Autodesk Inventor part; units mm, degrees
ref_plane "YZ Plane" through (0, 0, 0) normal (1, 0, 0) x (0, 1, 0)
ref_plane "XZ Plane" through (0, 0, 0) normal (0, 1, 0) x (-1, 0, 0)
ref_plane "XY Plane" through (0, 0, 0) normal (0, 0, 1) x (1, 0, 0)
sketch "Sketch1" plane through (0, 0, 0) normal (0, 1, 0) x (-1, 0, 0)
  line L0 (0, 0) -> (-88.9, 0)
  line L1 (-88.9, -114.3) -> (-88.9, -317.5)
  line L2 (-88.9, -431.8) -> (0, -431.8)
  line L3 (0, -431.8) -> (0, 0)
  line L4 (-88.9, 0) -> (-165.1, 0)
  line L5 (-165.1, 0) -> (-165.1, -114.3)
  line L6 (-165.1, -114.3) -> (-88.9, -114.3)
  line L7 (-88.9, -114.3) -> (-88.9, 0)
  line L8 (-88.9, -431.8) -> (-165.1, -431.8)
  line L9 (-165.1, -431.8) -> (-165.1, -317.5)
  line L10 (-165.1, -317.5) -> (-88.9, -317.5)
  line L11 (-88.9, -317.5) -> (-88.9, -431.8)
  line L12 (-88.9, -374.65) -> (-139.7, -374.65) construction
  line L13 (-88.9, -58.8342) -> (-139.7, -58.8342) construction
  circle A0 centre (-139.7, -58.8342) radius 7.9375
  circle A1 centre (-139.7, -374.65) radius 7.9375
  dimension "d0" = 88.9
  dimension "d1" = 431.8
  dimension "d2" = 76.2
  dimension "d3" = 114.3
  dimension "d4" = 76.2
  dimension "d5" = 114.3
  dimension "d6" = 50.8
  dimension "d7" = 15.875
  dimension "d8" = 15.875
extrude "Extrusion1" add sketch "Sketch1" along normal blind 6.35
sketch "Sketch8" plane through (0, 6.35, 0) normal (0, 1, 0) x (1, 0, 0)
  circle A0 centre (139.7, 58.8342) radius 7.9375
  circle A1 centre (139.7, 374.65) radius 7.9375
  line L0 (88.9, 317.5) -> (165.1, 317.5)
  line L1 (165.1, 317.5) -> (165.1, 431.8)
  line L2 (165.1, 431.8) -> (0, 431.8)
  line L3 (0, 431.8) -> (0, 0)
  line L4 (0, 0) -> (165.1, 0)
  line L5 (165.1, 0) -> (165.1, 114.3)
  line L6 (165.1, 114.3) -> (88.9, 114.3)
  line L7 (88.9, 114.3) -> (88.9, 317.5)
  line L8 (165.1, 0) -> (88.9, 0)
  line L9 (88.9, 0) -> (88.9, 3.175)
  line L10 (88.9, 3.175) -> (165.1, 3.175)
  line L11 (165.1, 3.175) -> (165.1, 0)
  line L12 (165.1, 114.3) -> (88.9, 114.3)
  line L13 (88.9, 114.3) -> (88.9, 111.125)
  line L14 (88.9, 111.125) -> (165.1, 111.125)
  line L15 (165.1, 111.125) -> (165.1, 114.3)
  line L16 (88.9, 114.3) -> (88.9, 317.5)
  line L17 (165.1, 317.5) -> (88.9, 317.5)
  line L18 (88.9, 317.5) -> (88.9, 320.675)
  line L19 (88.9, 320.675) -> (165.1, 320.675)
  line L20 (165.1, 320.675) -> (165.1, 317.5)
  line L21 (165.1, 431.8) -> (88.9, 431.8)
  line L22 (88.9, 431.8) -> (88.9, 428.625)
  line L23 (88.9, 428.625) -> (165.1, 428.625)
  line L24 (165.1, 428.625) -> (165.1, 431.8)
  dimension "d27" = 3.175
  dimension "d28" = 3.175
  dimension "d29" = 3.175
  dimension "d30" = 3.175
extrude "Extrusion7" add sketch "Sketch8" along normal blind 82.55 contours L18 L19 L1 L0 | L6 L5 L14 L13 | L23 L22 L2 L1 | L5 L4 L9 L10
sketch "Sketch9" plane through (165.1, 6.35, -3.175) normal (0, 0, -1) x (-1, 0, 0)
  line L0 (76.2, 0) -> (0, 0)
  line L1 (76.2, 0) -> (76.2, 82.55)
  line L2 (0, 82.55) -> (76.2, 82.55)
  line L3 (0, 0) -> (0, 82.55)
  line L4 (0, -6.35) -> (0, 82.55)
  line L5 (76.2, 82.55) -> (0, 82.55)
  line L6 (0, 82.55) -> (0, 76.2)
  line L7 (0, 76.2) -> (76.2, 76.2)
  line L8 (76.2, 76.2) -> (76.2, 82.55)
  point P0 (165.1, -6.35)
  dimension "d33" = 6.35
sketch "Sketch10" plane through (165.1, 6.35, -320.675) normal (0, 0, -1) x (-1, 0, 0)
  line L0 (76.2, -6.35) -> (0, -6.35)
  line L1 (0, -6.35) -> (0, 82.55)
  line L2 (76.2, 82.55) -> (0, 82.55)
  line L3 (76.2, 0) -> (76.2, 82.55)
  line L4 (76.2, -6.35) -> (76.2, 0)
  line L5 (0, 0) -> (0, 82.55)
  line L6 (76.2, 82.55) -> (0, 82.55)
  line L7 (0, 82.55) -> (0, 76.2)
  line L8 (0, 76.2) -> (76.2, 76.2)
  line L9 (76.2, 76.2) -> (76.2, 82.55)
  point P0 (165.1, -6.35)
  dimension "d34" = 6.35
extrude "Extrusion8" add sketch "Sketch9" along normal blind 107.95 contours L7 L3 L2 L1
extrude "Extrusion9" add sketch "Sketch10" along normal blind 107.95 contours L8 L1 L2 L3
sketch "Sketch11" plane through (88.9, 82.55, -320.675) normal (0, -1, 0) x (1, 0, 0)
  line L0 (0, 0) -> (76.2, 0)
  circle A0 centre (50.8, -53.975) radius 7.9375
  line L1 (0, 206.375) -> (0, 3.175)
  line L2 (76.2, -111.125) -> (-88.9, -111.125)
  line L3 (76.2, 3.175) -> (76.2, -111.125)
  line L4 (0, 3.175) -> (76.2, 3.175)
  circle A1 centre (50.8, 261.8408) radius 7.9375
  line L5 (0, 206.375) -> (0, 3.175)
  line L6 (76.2, 206.375) -> (0, 206.375)
  line L7 (76.2, 320.675) -> (76.2, 206.375)
  line L8 (-88.9, 320.675) -> (76.2, 320.675)
  line L9 (-88.9, -111.125) -> (-88.9, 320.675)
  line L10 (76.2, -111.125) -> (-88.9, -111.125)
  circle A2 centre (50.8, 261.8408) radius 7.9375
  circle A3 centre (50.8, -53.975) radius 7.9375
  circle A4 centre (50.8, 261.8408) radius 7.9375
  line L11 (76.2, 3.175) -> (76.2, -111.125)
  line L12 (0, 3.175) -> (76.2, 3.175)
  line L13 (76.2, 206.375) -> (0, 206.375)
  line L14 (76.2, 320.675) -> (76.2, 206.375)
  line L15 (-88.9, 320.675) -> (76.2, 320.675)
  line L16 (-88.9, -111.125) -> (-88.9, 320.675)
extrude "Extrusion10" cut sketch "Sketch11" against normal blind 25.4 contours A0
sketch "Sketch12" plane through (88.9, 82.55, -3.175) normal (0, -1, 0) x (1, 0, 0)
  circle A0 centre (50.8, -55.6592) radius 7.9375
  circle A1 centre (50.8, -55.6592) radius 7.9375
  point P0 (-88.9, 3.175)
extrude "Extrusion11" cut sketch "Sketch12" against normal blind 25.4
properties part number "side"
Can you work these out from the model? Positions are in its coordinate system, mm. A direction names the side the tool comes from. Give positions to 0.01 mm unless a question says otherwise; leave off trailing zeros. Order: outer loops, then holes, each group sorted by start corner. A loop starts at its lowest first (then second) coordinate and runs counter-clockwise, first axis right, second up. Notation, with made-up numbers: (43, 88.5) - (50, 88.5) arc R32 ccw to (50, 117.5) - close; hole circle Ø6 at (64, 89.25). An arc over 180 degrees is marked (long way). Write each question's results on one line, items separated by ' | '.
1) Suppose I cut it at C-C, the plane y = 59. Write out the boundary of the cut face in (x, z) (3 decimals), then the cut area to 3 significant figures.
Final values:
outline: (88.9, -431.8) - (165.1, -431.8) - (165.1, -428.625) - (88.9, -428.625) - close; (88.9, -320.675) - (165.1, -320.675) - (165.1, -317.5) - (88.9, -317.5) - close; (88.9, -114.3) - (165.1, -114.3) - (165.1, -111.125) - (88.9, -111.125) - close; (88.9, -3.175) - (165.1, -3.175) - (165.1, 0) - (88.9, 0) - close | area: 968 mm^2
2) On a 3-axis mill with a long thin cutter (end or side, diameter ignored), from which of +Z, -Z, +X, -X, +Y, -Y can I reach the whole of each face in a straight line? I mean faces 1 (the face through (165.1, 5, -370)), 2 (the face through (88.9, 84, -374)), 3 (the face through (126, 44, -111.125)). Say none if no direction works.
Final values:
face 1: +Z, -Z, +X, +Y, -Y | face 2: +Z, -Z, -X, +Y | face 3: +X, -X
3) If we mould it in two halves opening along Z, with no side actions, what happens to faces 4 (the face through (165.1, 5, -53)), 5 (the face through (120, 44, -431.8)), 6 (the face through (128, 44, -114.3))? For each: pulls with the +Z half, pulls with the -Z half, needs draft (parallel to the pull), parting line crosses it, or undercut.
Final values:
face 4: needs draft | face 5: pulls with the -Z half | face 6: undercut
4) Please list where these lines run through material, in increasing order: line 1 along Z through (x, y) = (99.5, 69.5) (3 decimals); line 2 along Z through (x, y) = (139.7, 85.25); line 3 along Y through (x, z) = (133.5, -385). Write a range as [from, to].
Final values:
line 1: z = [-431.8, -428.625], [-320.675, -317.5], [-114.3, -111.125], [-3.175, 0] | line 2: z = [-431.8, -382.59], [-366.71, -317.5], [-114.3, -66.77], [-50.9, 0] | line 3: y = [0, 6.35], [82.55, 88.9]
5) Suppose I cut it at B-B, the plane z = -374.65. Write out the boundary of the cut face in (x, y), then the cut area to 3 significant figures.
Final values:
outline: (0, 0) - (131.76, 0) - (131.76, 6.35) - (0, 6.35) - close; (88.9, 82.55) - (131.76, 82.55) - (131.76, 88.9) - (88.9, 88.9) - close; (147.64, 0) - (165.1, 0) - (165.1, 6.35) - (147.64, 6.35) - close; (147.64, 82.55) - (165.1, 82.55) - (165.1, 88.9) - (147.64, 88.9) - close | area: 1,330 mm^2
6) Suppose I cut it at D-D, the plane x = 139.7. Give the number of separate pieces and of enclosed holes in the cut face, then the cut area to 3 significant figures.
Final values:
separate pieces: 4 | enclosed holes: 0 | area: 3,470 mm^2
7) Suppose I cut it at A-A, the plane x = 103. Write out the boundary of the cut face in (y, z) (3 decimals), then the cut area to 3 significant figures.
Final values:
outline: (0, -431.8) - (88.9, -431.8) - (88.9, -317.5) - (0, -317.5) - close; (0, -114.3) - (88.9, -114.3) - (88.9, 0) - (0, 0) - close; hole (6.35, -428.625) - (82.55, -428.625) - (82.55, -320.675) - (6.35, -320.675) - close; hole (6.35, -111.125) - (82.55, -111.125) - (82.55, -3.175) - (6.35, -3.175) - close | area: 3,870 mm^2
